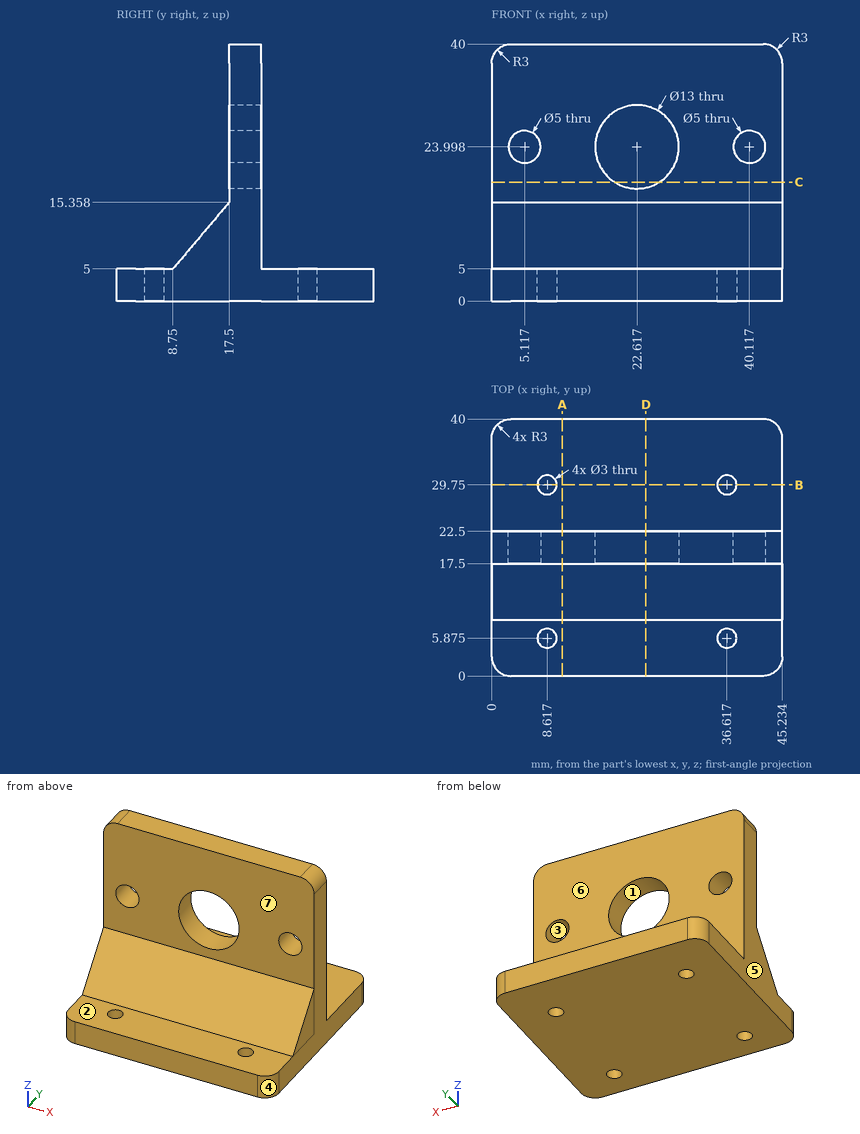
Could you check a few things on this drawing? It's one solid part, dimensions in mm from its lowest x, y, z. A direction names the side the tool comes from. Give positions to 0.01 mm unless a question says otherwise; leave off trailing zeros. Write each loop counter-clockwise with the first axis right and the second up, starting at its lowest first coordinate (ties: lowest second). Pieces come first, ordered by that corner, then holes.
(1) Will these pins go through, and if not, where does the flat tip stop? pin 1 (8 mm diameter, centred on x = 5.12, z = 24, fed in from -Y); pin 2 (4 mm diameter, centred on x = 8.62, y = 5.88, fed in from +Z); pin 3 (12 mm diameter, centred on x = 20.5, z = 13.5, fed in from -Y).
Output values:
pin 1: stops at y = 17.5
pin 2: stops at z = 5
pin 3: stops at y = 10.86
(2) Imagine slicing it at D-D, the plane x = 24. Write out the boundary of the cut face in (y, z), and give its area (3 significant figures).
Output values:
outline: (0, 0) - (40, 0) - (40, 5) - (22.5, 5) - (22.5, 17.65) - (17.5, 17.65) - (17.5, 15.36) - (8.75, 5) - (0, 5) - close; (17.5, 30.35) - (22.5, 30.35) - (22.5, 40) - (17.5, 40) - close
area: 357 mm2
(3) On a 3-axis mill with a long thin cutter (end or side, diameter ignored), from which of +Z, -Z, +X, -X, +Y, -Y can I reach the whole of each face in a straight line? I mean the marked faces 5, 6 and 7. Say none if no direction works.
Output values:
face 5: +Z, -Z, -X, +Y, -Y
face 6: +Z, +X, -X, +Y
face 7: +Z, +X, -X, -Y
(4) Imagine slicing it at C-C, the plane z = 18.5. Write out the boundary of the cut face in (x, y) (1 decimal).
Output values:
outline: (0, 17.5) - (19.1, 17.5) - (19.1, 22.5) - (0, 22.5) - close; (26.1, 17.5) - (45.2, 17.5) - (45.2, 22.5) - (26.1, 22.5) - close
(5) Thinking about a two-plate mould opening in X: for the marked faces 1, 2, 3 and 4, which applies, pulls with the +X half, pulls with the -X half, needs draft (parallel to the pull), parting line crosses it, or undercut?
Output values:
face 1: undercut
face 2: needs draft
face 3: undercut
face 4: pulls with the +X half
(6) Imagine slicing it at A-A, the plane x = 11. Write out the boundary of the cut face in (y, z), and give its area (3 significant figures).
Output values:
outline: (0, 0) - (40, 0) - (40, 5) - (22.5, 5) - (22.5, 40) - (17.5, 40) - (17.5, 15.36) - (8.75, 5) - (0, 5) - close
area: 420 mm2
(7) If I drill on L1, parallel to Z at x = 11.5, y = 35; L2, parallel to Y at x = 10, z = 22; L3, parallel to Y at x = 42.5, z = 12.5 (1 decimal), over which ranges is the centre line in solid material (lowest first)?
Output values:
L1: z = 0 to 5
L2: y = 17.5 to 22.5
L3: y = 15.1 to 22.5
(8) Imagine slicing it at B-B, the plane y = 29.75. Write out the boundary of the cut face in (x, z).
Output values:
outline: (0, 0) - (7.12, 0) - (7.12, 5) - (0, 5) - close; (10.12, 0) - (35.12, 0) - (35.12, 5) - (10.12, 5) - close; (38.12, 0) - (45.23, 0) - (45.23, 5) - (38.12, 5) - close
